Can you work these out from the model? Positions are in its coordinate system, mm. Face numbers are marked on the shaded views. Coordinates: 2 decimals unless noted, no trailing zeros. Order: outer loops, then holes, each group sorted by start corner. A loop starts at its lowest first (then second) coordinate and runs counter-clockwise, first axis right, second up. Notation, with made-up numbers: (74, 81.25) -> (96, 81.25) arc R23 cw to (96, 103.25) -> close; hole circle Ø8 at (1.25, -23). An arc over 180 degrees is marked (long way). Answer as a JSON object with one key per item and string values. Group by question number.
(1) If we mould it in two halves opening along Z, with no side actions, what happens to the marked faces 1, 2 and 3? For each: pulls with the +Z half, pulls with the -Z half, needs draft (parallel to the pull), parting line crosses it, or undercut.
(2) I want a section at B-B, the plane z = -8.25. List the corners of the cut face in (x, y) for me.
(3) I want a section at A-A, the plane z = 2.5. List the corners of the cut face in (x, y) for me.
(4) I need wall thicknesses on line 1 (X direction, y = -0.65, z = 7.5); line 2 (X direction, y = -0.9, z = 6.5); line 3 (X direction, y = -0.1, z = -5.25). Which ranges of each line are inside material? Lowest first, please.
(5) I want a section at C-C, the plane y = -1.4. State how many separate pieces and enclosed holes the cut face has, plus the area to 3 significant figures.
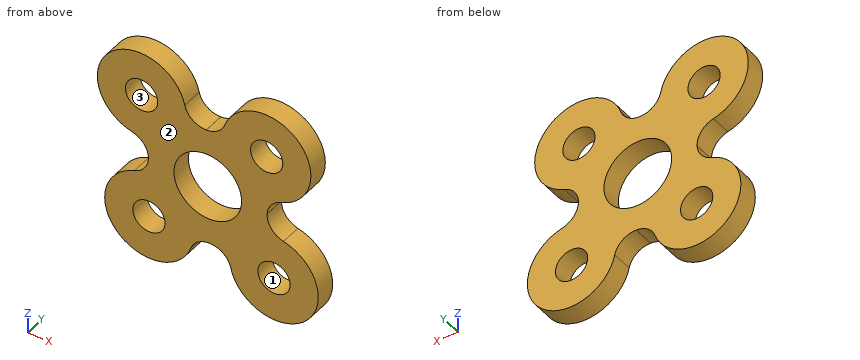
from build123d import *

# Parameters (mm, degrees)
SKETCH1_R           = 1.55
SKETCH1_R_2         = 3.25
BOSS_EXTRUDE2_DEPTH = 2
FILLET1_R           = 2


with BuildPart() as part:
    # Sketch1 → Boss-Extrude2 (new body)
    with BuildSketch(Plane(origin=(0, 0, 0), x_dir=(1, 0, 0), z_dir=(0, 1, 0))):
        with BuildLine():
            ThreePointArc((-1.43909166, 6.179327925), (-8.65976943, 8.664344967), (-6.18574902, 1.439892035))
            ThreePointArc((-6.18574902, 1.439892035), (-5.7, -0.338953386), (-6.18574902, -2.117798807))
            ThreePointArc((-6.18574902, -2.117798807), (-9.366987419, -9.371531966), (-2.118073304, -6.179327925))
            ThreePointArc((-2.118073304, -6.179327925), (-0.339490822, -5.693734061), (1.43909166, -6.179327925))
            ThreePointArc((1.43909166, -6.179327925), (8.65976943, -8.664344967), (6.18574902, -1.439892035))
            ThreePointArc((6.18574902, -1.439892035), (5.7, 0.338953386), (6.18574902, 2.117798807))
            ThreePointArc((6.18574902, 2.117798807), (9.366987419, 9.371531966), (2.118073304, 6.179327925))
            ThreePointArc((2.118073304, 6.179327925), (0.339490822, 5.693734061), (-1.43909166, 6.179327925))
        make_face()
        with Locations(Location((-6.364056731, -6.364056731, 0), (0, 0, 270))):
            Circle(SKETCH1_R, mode=Mode.SUBTRACT)
        with Locations(Location((6.364056731, 6.364056731, 0), (0, 0, 270))):
            Circle(SKETCH1_R, mode=Mode.SUBTRACT)
        with Locations(Location((5.656854249, -5.656854249, 0), (0, 0, 270))):
            Circle(SKETCH1_R, mode=Mode.SUBTRACT)
        with Locations(Location((-5.656854249, 5.656854249, 0), (0, 0, 270))):
            Circle(SKETCH1_R, mode=Mode.SUBTRACT)
        with Locations(Location((0, 0, 0), (0, 0, 270))):
            Circle(SKETCH1_R_2, mode=Mode.SUBTRACT)
    extrude(amount=-BOSS_EXTRUDE2_DEPTH)

    # Fillet1
    fillet1_edges = [part.edges().sort_by_distance(p)[0] for p in [
        (-2.118073304, -1, 6.179327925),
        (-6.18574902, -1, 2.117798807),
        (-6.18574902, -1, -1.439892035),
        (-1.43909166, -1, -6.179327925),
        (2.118073304, -1, -6.179327925),
        (6.18574902, -1, -2.117798807),
        (6.18574902, -1, 1.439892035),
        (1.43909166, -1, 6.179327925),
    ]]
    fillet(fillet1_edges, radius=FILLET1_R)


solid = part.part
Computed values:
{
 "1": {"face 1": "undercut", "face 2": "needs draft", "face 3": "undercut"},
 "2": {"outline": "(-9.02, -2) -> (-2.29, -2) -> (-2.29, 0) -> (-9.02, 0) -> close; (2.56, -2) -> (10.17, -2) -> (10.17, 0) -> (2.56, 0) -> close"},
 "3": {"outline": "(-8.13, -2) -> (-2.08, -2) -> (-2.08, 0) -> (-8.13, 0) -> close; (2.08, -2) -> (8.5, -2) -> (8.5, 0) -> (2.08, 0) -> close"},
 "4": {"line 1": "x = -10.46 to -7.42, -5.31 to -2.27, 1.83 to 9.49", "line 2": "x = -10.61 to -7.91, -4.82 to -1.86, 1.35 to 4.36, 6.96 to 9.82", "line 3": "x = -9.89 to -7.15, -4.16 to 5.29, 7.44 to 10.47"},
 "5": {"separate pieces": "1", "enclosed holes": "5", "area": "251 mm2"}
}
